For this review, use the dimensioned drawing (mm, ordinates from the lowest corner) and the shaded views. Round coordinates to 2 decimals unless told otherwise and drop trailing zeros. Loops run counter-clockwise (first coordinate to the right, second up) from the corner with the lowest first, then second, coordinate; pieces in that order, holes last. Notation, with made-up numbers: M 23,-0.5 L 38,-0.5 A12 ccw 38,6.5 Z; hole C 47,88 d10. An arc over 180 degrees is marked long. Answer as a JSON object with one key per item and string values. Group by question number.
Item 1: Consider section A-A (z = 14.2). Give the boundary of the cut face in (x, y) (3 decimals).
Item 2: To check wall thickness, follow line 1 (X direction, y = 0.75, z = 6.25); line 2 (X direction, y = 0.2, z = 24); line 3 (Z direction, x = 5.5, y = 1.45) (3 decimals). State the ranges of each line that lie inside material, in increasing order.
Item 3: Insertion check: P1, Ø2.5, axis at x = 25.375, z = 14.2, coming from the -Y side; P2, Ø0.6, axis at x = 7, y = 1, coming from the +Z side. Each pin has a flat end and moves straight along its axis. Give the tip position at first contact, or say it passes through.
Item 4: Consider section B-B (x = 6). Give the boundary of the cut face in (y, z) (3 decimals).
Item 5: Consider section D-D (y = 1.65). State how many separate pieces and enclosed holes the cut face has, and give its area (3 significant figures).
Item 6: Consider section C-C (x = 27.5). Give the boundary of the cut face in (y, z), and give its area (3 significant figures).
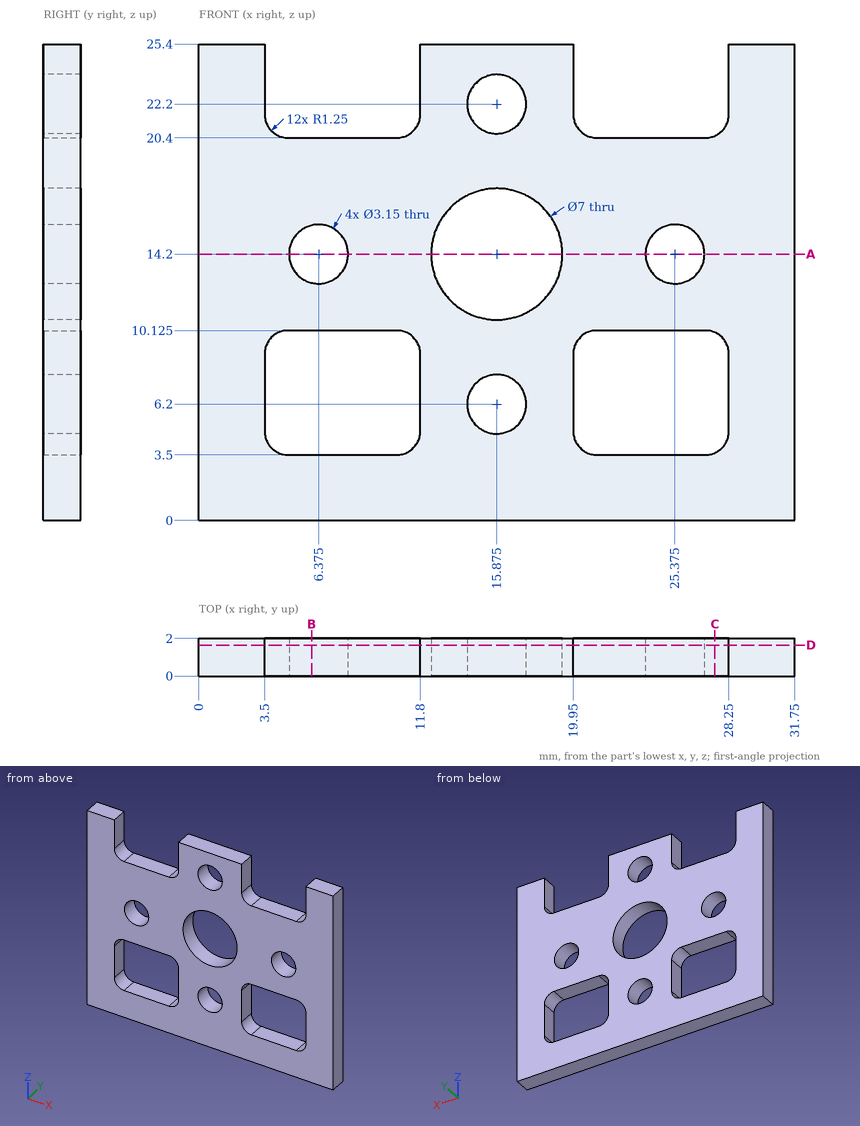
Geometry results:
{
 "1": {"outline": "M 0,0 L 4.8,0 L 4.8,2 L 0,2 Z; M 7.95,0 L 12.375,0 L 12.375,2 L 7.95,2 Z; M 19.375,0 L 23.8,0 L 23.8,2 L 19.375,2 Z; M 26.95,0 L 31.75,0 L 31.75,2 L 26.95,2 Z"},
 "2": {"line 1": "x = 0 to 3.5, 11.8 to 14.3, 17.45 to 19.95, 28.25 to 31.75", "line 2": "x = 0 to 3.5, 11.8 to 19.95, 28.25 to 31.75", "line 3": "z = 0 to 3.5, 10.125 to 12.89, 15.51 to 20.4"},
 "3": {"P1": "passes through", "P2": "stops at z = 20.4"},
 "4": {"outline": "M 0,0 L 2,0 L 2,3.5 L 0,3.5 Z; M 0,10.125 L 2,10.125 L 2,12.67 L 0,12.67 Z; M 0,15.73 L 2,15.73 L 2,20.4 L 0,20.4 Z"},
 "5": {"separate pieces": "1", "enclosed holes": "7", "area": "548 mm^2"},
 "6": {"outline": "M 0,0 L 2,0 L 2,3.6 L 0,3.6 Z; M 0,10.02 L 2,10.02 L 2,20.5 L 0,20.5 Z", "area": "28.2 mm^2"}
}
